```python
from build123d import *

# Parameters (mm, degrees)
SKETCH_4_W          = 23.255
SKETCH_4_H          = 57.4134
SKETCH_4_R          = 0.6
EXTRUDE_5_DEPTH     = 4
SKETCH_5_W          = 65.55
SKETCH_5_H          = 20.755
SKETCH_5_R          = 1.55
EXTRUDE_6_DEPTH     = 4
SKETCH_7_W          = 65.55
SKETCH_7_H          = 126.45
EXTRUDE_8_DEPTH     = 4
SKETCH_11_W         = 17.25
SKETCH_11_H         = 32.3
SKETCH_11_W_2       = 18.8
SKETCH_11_H_2       = 10.8
CUT_EXTRUDE_3_DEPTH = 125.085535116
EXTRUDE_9_DEPTH     = 4
CUT_EXTRUDE_4_DEPTH = 10
SKETCH_14_W         = 9.75
SKETCH_14_H         = 12.755
CUT_EXTRUDE_5_DEPTH = 10
SKETCH_16_W         = 15.255
SKETCH_16_H         = 24.775
SKETCH_16_W_2       = 15.505
SKETCH_16_H_2       = 9.88
CUT_EXTRUDE_6_DEPTH = 133.101854737
SKETCH_17_R         = 0.875
EXTRUDE_10_DEPTH    = 1
FILLET_1_R          = 0.5
EXTRUDE_2_DEPTH     = 4
CUT_EXTRUDE_7_REACH = 127.473
SKETCH_19_R         = 1.1
SKETCH_21_W         = 4
SKETCH_21_H         = 2.5
EXTRUDE_11_DEPTH    = 4
FILLET_2_R          = 2
FILLET_3_R          = 4.65


with BuildPart() as part:
    # 草图4 → 凸台-拉伸5 (new body)
    with BuildSketch(Plane(origin=(37.65, 0, 0), x_dir=(0, 0, -1), z_dir=(1, 0, 0))):
        with Locations((11.6275, 81.8433)):
            Rectangle(SKETCH_4_W, SKETCH_4_H)
        with Locations(Location((10.735, 94.05, 0), (0, 0, 90))):
            Circle(SKETCH_4_R, mode=Mode.SUBTRACT)
        with Locations(Location((10.735, 57.65, 0), (0, 0, 90))):
            Circle(SKETCH_4_R, mode=Mode.SUBTRACT)
    extrude(amount=EXTRUDE_5_DEPTH)

    # 草图5 → 凸台-拉伸6 (add)
    with BuildSketch(Plane(origin=(0, 110.55, 0), x_dir=(1, 0, 0), z_dir=(0, 1, 0))):
        with Locations((8.875, 10.3775)):
            Rectangle(SKETCH_5_W, SKETCH_5_H)
        with Locations(Location((-18.9, 15.755, 0), (0, 0, 180))):
            Circle(SKETCH_5_R, mode=Mode.SUBTRACT)
        with Locations(Location((18.9, 15.755, 0), (0, 0, 180))):
            Circle(SKETCH_5_R, mode=Mode.SUBTRACT)
    extrude(amount=EXTRUDE_6_DEPTH)

    # 草图7 → 凸台-拉伸8 (add)
    with BuildSketch(Plane.XY):
        with Locations((8.875, 51.325)):
            Rectangle(SKETCH_7_W, SKETCH_7_H)
    extrude(amount=EXTRUDE_8_DEPTH)

    # 草图11 → 切除-拉伸3 (cut, through all)
    with BuildSketch(Plane(origin=(0, 0, 0), x_dir=(-1, 0, 0), z_dir=(0, 0, -1))):
        with Locations((-25.025, 12.25)):
            Rectangle(SKETCH_11_W, SKETCH_11_H)
        Polygon((-33.65, 106.55), (-33.65, 36.4), (-16.4, 36.4), (8.4, 36.4), (8.4, 106.55), align=None)
        with Locations((-1, 1.5)):
            Rectangle(SKETCH_11_W_2, SKETCH_11_H_2)
        with Locations((-1, 23)):
            Rectangle(SKETCH_11_W_2, SKETCH_11_H_2)
        with BuildLine():
            ThreePointArc((16.4, -7.25), (15.038046533, -10.538046533), (11.75, -11.9))
            Line((11.75, -11.9), (23.9, -11.9))
            Line((23.9, -11.9), (23.9, 106.55))
            Line((23.9, 106.55), (16.4, 106.55))
            Line((16.4, 106.55), (16.4, -7.25))
        make_face()
    extrude(amount=-CUT_EXTRUDE_3_DEPTH, mode=Mode.SUBTRACT)

    # 草图12 → 凸台-拉伸9 (add)
    with BuildSketch(Plane(origin=(0, 2.890336251, 0), x_dir=(1, 0, 0), z_dir=(0, 1, 0))):
        with BuildLine():
            Line((46.295757056, 9.855), (50.995757056, 9.855))
            Line((50.995757056, 9.855), (50.995757056, 15.105))
            Line((50.995757056, 15.105), (49.455691264, 15.105))
            ThreePointArc((49.455691264, 15.105), (47.695757056, 15.755), (49.455691264, 16.405))
            Line((49.455691264, 16.405), (50.995757056, 16.405))
            Line((50.995757056, 16.405), (50.995757056, 21.655))
            Line((50.995757056, 21.655), (46.295757056, 21.655))
            Line((46.295757056, 21.655), (46.295757056, 9.855))
        make_face()
        Polygon((52.295757056, 6.645757056), (52.295757056, 9.855), (50.995757056, 9.855), (46.295757056, 9.855), (36.440757056, 0), (41.65, -4), align=None)
        with BuildLine():
            Line((52.295757056, 9.855), (52.295757056, 21.655))
            Line((52.295757056, 21.655), (50.995757056, 21.655))
            Line((50.995757056, 21.655), (50.995757056, 16.405))
            Line((50.995757056, 16.405), (49.455691264, 16.405))
            ThreePointArc((49.455691264, 16.405), (47.695757056, 15.755), (49.455691264, 15.105))
            Line((49.455691264, 15.105), (50.995757056, 15.105))
            Line((50.995757056, 15.105), (50.995757056, 9.855))
            Line((50.995757056, 9.855), (52.295757056, 9.855))
        make_face()
    extrude(amount=EXTRUDE_9_DEPTH)

    # 草图13 → 切除-拉伸4 (cut, symmetric)
    with BuildSketch(Plane.XZ.offset(-110.55)):
        Polygon((-23.9, -7.5), (-16.4, 0), (-16.4, 4), (-23.9, 4), align=None)
    extrude(amount=CUT_EXTRUDE_4_DEPTH, both=True, mode=Mode.SUBTRACT)

    # 草图14 → 切除-拉伸5 (cut)
    with BuildSketch(Plane.XZ.offset(-110.55)):
        with Locations((28.775, -10.3775)):
            Rectangle(SKETCH_14_W, SKETCH_14_H)
        Polygon((13.9, -16.755), (-13.9, -16.755), (-13.9, -11.642135624), (-6.257864376, -4), (13.9, -4), align=None)
    extrude(amount=-CUT_EXTRUDE_5_DEPTH, mode=Mode.SUBTRACT)

    # 草图16 → 切除-拉伸6 (cut, through all)
    with BuildSketch(Plane.ZY.offset(-37.65)):
        with Locations((-11.6275, 76.6625)):
            Rectangle(SKETCH_16_W, SKETCH_16_H)
        with Locations((-11.5025, 105.61)):
            Rectangle(SKETCH_16_W_2, SKETCH_16_H_2)
    extrude(amount=-CUT_EXTRUDE_6_DEPTH, mode=Mode.SUBTRACT)

    # 草图17 → 凸台-拉伸10 (add)
    with BuildSketch(Plane.ZY.offset(-37.65)):
        with Locations(Location((-10.735, 62.275, 0), (0, 0, 90))):
            Circle(SKETCH_17_R)
        with BuildLine():
            Line((-11.635, 97.922403852), (-11.635, 99.417596148))
            ThreePointArc((-11.635, 99.417596148), (-10.735, 99.84), (-9.835, 99.417596148))
            Line((-9.835, 99.417596148), (-9.835, 97.922403852))
            ThreePointArc((-9.835, 97.922403852), (-10.735, 97.5), (-11.635, 97.922403852))
        make_face()
    extrude(amount=EXTRUDE_10_DEPTH)

    # 圆角1
    # the kernel refuses this fillet: 0.5 mm, written as the material it takes off along each edge
    with BuildSketch(Plane(origin=(36.65, 62.275, -10.735), x_dir=(0, 1, 0), z_dir=(0, 0, 1))) as fillet_1_piece_1:
        with BuildLine():
            CenterArc((0.875 - FILLET_1_R, -FILLET_1_R), FILLET_1_R, 0, 90)
            Line((0.875 - FILLET_1_R, 0), (0.875, 0))
            Line((0.875, 0), (0.875, -FILLET_1_R))
        make_face()
    revolve(axis=Axis((36.65, 62.275, -10.735), (-1, 0, 0)), mode=Mode.SUBTRACT)
    with BuildSketch(Plane(origin=(36.65, 96.672403852, -11.635), x_dir=(1, 0, 0), z_dir=(0, 1, 0)), Plane(origin=(36.65, 100.667596148, -9.835), x_dir=(1, 0, 0), z_dir=(0, -1, 0))) as fillet_1_piece_2:
        with BuildLine():
            CenterArc((FILLET_1_R, -FILLET_1_R), FILLET_1_R, 90, 90)
            Line((0, -FILLET_1_R), (0, 0))
            Line((0, 0), (FILLET_1_R, 0))
        make_face()
    extrude(amount=3.995192295, mode=Mode.SUBTRACT)
    with BuildSketch(Plane(origin=(36.65, 98.67, -10.735), x_dir=(0, 0.36697225923969184, 0.9302318855793519), z_dir=(0, 0.9302318855793519, -0.36697225923969184))) as fillet_1_piece_3:
        with BuildLine():
            CenterArc((1.17 - FILLET_1_R, FILLET_1_R), FILLET_1_R, 270, 90)
            Line((1.17 - FILLET_1_R, 0), (1.17, 0))
            Line((1.17, 0), (1.17, FILLET_1_R))
        make_face()
    revolve(axis=Axis((36.65, 98.67, -10.735), (1, 0, 0)), revolution_arc=223.058018827, mode=Mode.SUBTRACT)
    with BuildSketch(Plane(origin=(36.65, 98.67, -10.735), x_dir=(0, -0.36697225923969184, -0.9302318855793519), z_dir=(0, -0.9302318855793519, 0.36697225923969184))) as fillet_1_piece_4:
        with BuildLine():
            CenterArc((1.17 - FILLET_1_R, FILLET_1_R), FILLET_1_R, 270, 90)
            Line((1.17 - FILLET_1_R, 0), (1.17, 0))
            Line((1.17, 0), (1.17, FILLET_1_R))
        make_face()
    revolve(axis=Axis((36.65, 98.67, -10.735), (1, 0, 0)), revolution_arc=223.058018827, mode=Mode.SUBTRACT)

    # 草图2 → 凸台-拉伸2 (add)
    with BuildSketch(Plane.ZY.offset(16.4)):
        Polygon((-8, 12.25), (-8, 8.9), (4, 8.9), (4, 17.25), (-8, 17.25), align=None)
        with BuildLine():
            ThreePointArc((-2.75, 12.25), (-4, 11), (-5.25, 12.25))
            ThreePointArc((-5.25, 12.25), (-4, 13.5), (-2.75, 12.25))
        make_face(mode=Mode.SUBTRACT)
    extrude_2 = extrude(amount=EXTRUDE_2_DEPTH)

    # 镜向10: 凸台-拉伸2 across plane
    add(extrude_2.mirror(Plane(origin=(0, 0, 0), x_dir=(0, 0, 1), z_dir=(1, 0, 0))))

    # 草图19 → 切除-拉伸7 (cut, up to next)
    with BuildSketch(Plane.XZ.offset(-2.890336251), mode=Mode.PRIVATE) as cut_extrude_7_sk1:
        with Locations((48.695757056, -15.755)):
            Circle(SKETCH_19_R)
    cut_extrude_7_tool1 = extrude(cut_extrude_7_sk1.sketch, amount=-CUT_EXTRUDE_7_REACH, mode=Mode.PRIVATE) & part.part
    add(cut_extrude_7_tool1.solids().sort_by_distance((48.695757, 2.890336, -15.755))[0], mode=Mode.SUBTRACT)

    # 草图21 → 凸台-拉伸11 (add)
    with BuildSketch(Plane(origin=(0, 110.55, 0), x_dir=(1, 0, 0), z_dir=(0, 1, 0))):
        with Locations((39.65, 22.005)):
            Rectangle(SKETCH_21_W, SKETCH_21_H)
    extrude(amount=EXTRUDE_11_DEPTH)

    # 圆角2
    fillet_2_edges = [part.edges().sort_by_distance(p)[0] for p in [
        (33.65, 106.55, 2),
        (37.65, 110.55, -1.875),
        (37.65, 110.55, -20.005),
        (41.65, 114.55, -9.6275),
    ]]
    fillet(fillet_2_edges, radius=FILLET_2_R)

    # 圆角3
    fillet_3_edges = [part.edges().sort_by_distance(p)[0] for p in [
        (41.65, -11.9, 2),
    ]]
    fillet(fillet_3_edges, radius=FILLET_3_R)


solid = part.part
```
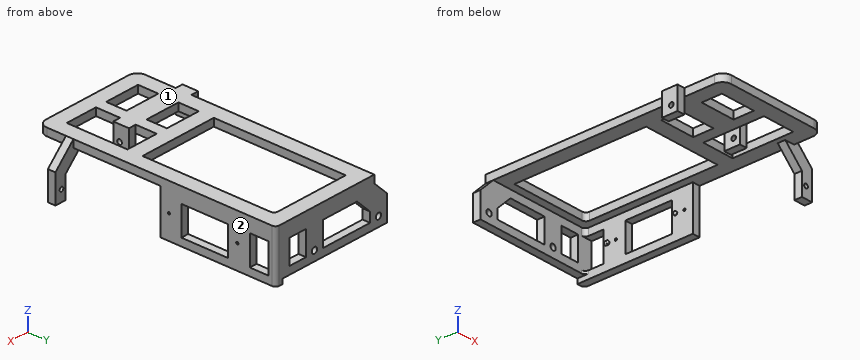
Check sheet for the modelled part. Datum: model origin and axes. Units: mm. Face numbers are marked on the shaded views. A direction names the side the tool comes from. Round coordinates to 2 decimals unless told otherwise and drop trailing zeros. Order: outer loops, then holes, each group sorted by start corner. A loop starts at its lowest first (then second) coordinate and runs counter-clockwise, first axis right, second up.
1) Section check C-C (y = 41). Record the boundary of the cut face in (x, z), and give its area (3 significant figures).
2) Section check A-A (x = 18.9). Record the boundary of the cut face in (y, z) (3 decimals), and give its area (3 significant figures).
3) Scan lines: line 1 (Y direction, x = -17.45, z = -4); line 2 (X direction, y = 86.5, z = 2); line 3 (Z direction, x = 18.9, y = 113.45) (3 decimals). Record each from-to range of solid material in increasing order.
4) Section check B-B (x = -18.9). Record the boundary of the cut face in (y, z) (3 decimals), and give its area (3 significant figures).
5) Tool access check on the marked faces 1 and 2. Record the directions out of +Z, -Z, +X, -X, +Y, -Y that give a thin tool (end or side, any length) a straight path to the whole face; none if there is none.
6) Go/stop test with flat-tipped pins: pin 1 Ø12 at (y, z) = (70, -8) entering from +X; pin 2 Ø4.5 at (x, y) = (6.5, 113) entering from -Z (3 decimals); pin 3 Ø5 at (x, z) = (35.5, -15.5) entering from -Y. Record where each tip stops, or that it passes through.
Result:
1. outline: (-16.4, 0) - (-8.4, 0) - (-8.4, 4) - (-16.4, 4) - close; (33.65, 0) - (41.65, 0) - (41.65, 4) - (33.65, 4) - close
1. area: 64.0 mm2
2. outline: (-11.9, 0) - (-3.9, 0) - (-3.9, 4) - (-11.9, 4) - close; (8.9, -8) - (17.25, -8) - (17.25, 4) - (8.9, 4) - close; (28.4, 0) - (36.4, 0) - (36.4, 4) - (28.4, 4) - close; (106.55, 0) - (110.55, 0) - (110.55, -14.205) - (114.55, -14.205) - (114.55, 4) - (106.55, 4) - close; (110.55, -20.755) - (114.55, -20.755) - (114.55, -17.305) - (110.55, -17.305) - close; hole circle Ø2.5 at (12.25, -4)
2. area: 262 mm2
3. line 1: y = 8.9 to 11, 13.5 to 17.25, 110.55 to 114.55
3. line 2: x = -16.4 to -8.4, 33.65 to 41.65
3. line 3: z = -20.755 to -17.305, -14.205 to 4
4. outline: (8.9, -8) - (17.25, -8) - (17.25, 4) - (8.9, 4) - close; (110.55, -20.755) - (114.55, -20.755) - (114.55, -17.305) - (110.55, -17.305) - close; (110.55, -14.205) - (114.55, -14.205) - (114.55, -2.5) - (110.55, -2.5) - close; hole circle Ø2.5 at (12.25, -4)
4. area: 156 mm2
5. face 1: +Z, +X, -X, +Y, -Y
5. face 2: +Z, -Z, +X, +Y
6. pin 1: stops at x = 41.65
6. pin 2: stops at z = -20.755
6. pin 3: stops at y = 53.14
